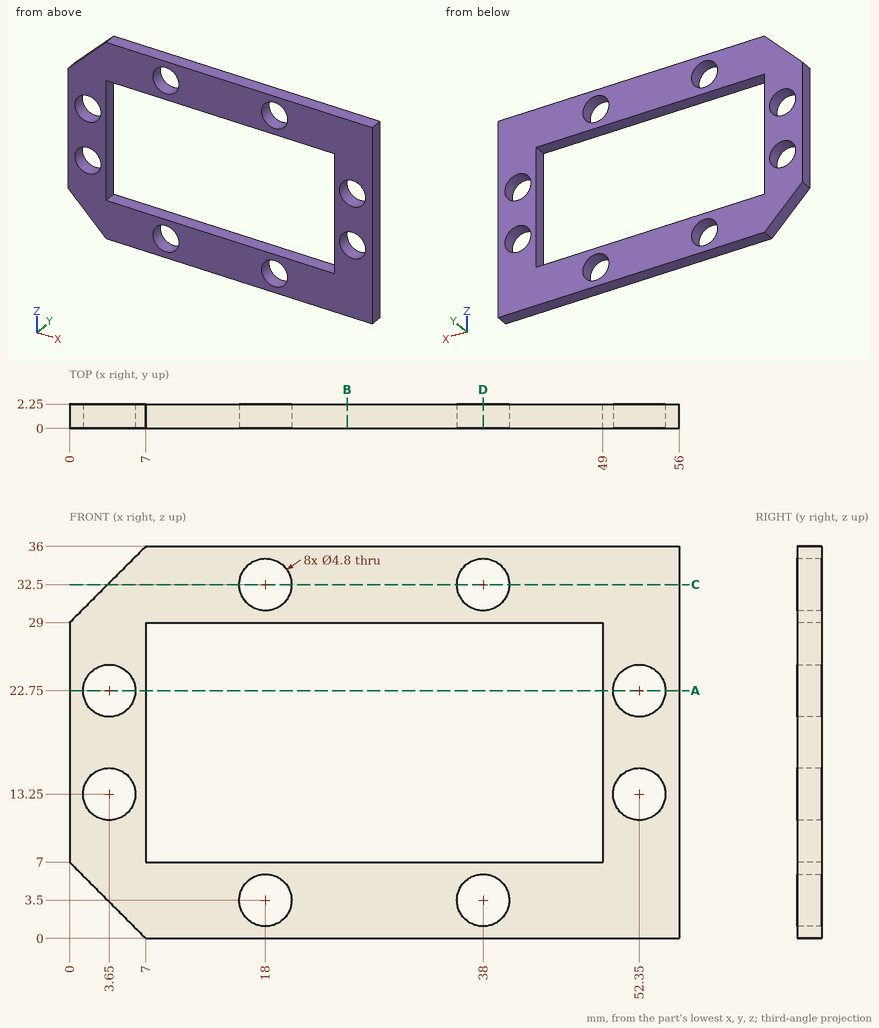
Geometry check sheet. Reference: drawing and pictorial views, mm from the part's lowest x, y, z. Round coordinates to 2 decimals unless told otherwise and drop trailing zeros. Loops run counter-clockwise (first coordinate to the right, second up) from the corner with the lowest first, then second, coordinate; pieces in that order, holes last. Notation, with made-up numbers: (54.5, -32) - (80.5, -32) arc R5 ccw to (80.5, -23) - close; hole circle Ø7 at (84.5, 56). An arc over 180 degrees is marked (long way). One line per question, with ' | ' between items. Start each with the question number.
1. Scan lines: line 1 (Z direction, x = 10.5, y = 1.5); line 2 (Z direction, x = 37.5, y = 1.8); line 3 (Z direction, x = 19, y = 1.1). Record each from-to range of solid material in increasing order. Write a range as [from, to].
2. Cross-section at C-C on z = 32.5. Record the cut outline in (x, y), then the cut area to 3 significant figures.
3. Cross-section at B-B on x = 25.5. Record the cut outline in (y, z).
4. Depth check by flat-ended pin: pin 1 (8 mm diameter, centred on x = 42.5, z = 25.5, fed in from +Y). Enter the tip coordinate at first touch or a pass-through.
5. Cross-section at D-D on x = 38. Record the cut outline in (y, z), then the cut area to 3 significant figures.
6. Cross-section at A-A on z = 22.75. Record the cut outline in (x, y).
Taken from the geometry:
1) line 1: [0, 7], [29, 36] | line 2: [0, 1.15], [5.85, 7], [29, 30.15], [34.85, 36] | line 3: [0, 1.32], [5.68, 7], [29, 30.32], [34.68, 36]
2) outline: (3.5, 0) - (15.6, 0) - (15.6, 2.25) - (3.5, 2.25) - close; (20.4, 0) - (35.6, 0) - (35.6, 2.25) - (20.4, 2.25) - close; (40.4, 0) - (56, 0) - (56, 2.25) - (40.4, 2.25) - close | area: 96.5 mm²
3) outline: (0, 0) - (2.25, 0) - (2.25, 7) - (0, 7) - close; (0, 29) - (2.25, 29) - (2.25, 36) - (0, 36) - close
4) pin 1: y = 2.25
5) outline: (0, 0) - (2.25, 0) - (2.25, 1.1) - (0, 1.1) - close; (0, 5.9) - (2.25, 5.9) - (2.25, 7) - (0, 7) - close; (0, 29) - (2.25, 29) - (2.25, 30.1) - (0, 30.1) - close; (0, 34.9) - (2.25, 34.9) - (2.25, 36) - (0, 36) - close | area: 9.90 mm²
6) outline: (0, 0) - (1.25, 0) - (1.25, 2.25) - (0, 2.25) - close; (6.05, 0) - (7, 0) - (7, 2.25) - (6.05, 2.25) - close; (49, 0) - (49.95, 0) - (49.95, 2.25) - (49, 2.25) - close; (54.75, 0) - (56, 0) - (56, 2.25) - (54.75, 2.25) - close
